For this review, take the finished solid that the model builds, in its own axes (mm). Give positions to 0.01 mm unless a question says otherwise; leave off trailing zeros. Use CSV: the item, a comma, the result in double quotes. Start each with the question number.
(1) Consider section A-A (y = -249.5). Give the number of separate pieces and of enclosed holes in the cut face, and give its area (3 significant figures).
(2) Clearance check with flat-ended pins moving along their axes: P1, Ø1.5, axis at x = 14.5, y = -333.5, coming from the -Z side; P2, Ø1.5, axis at y = -369, z = 14.5, coming from the -X side. State where each tip first meets the part, or that it passes through.
(3) Wall thickness on L1, parallel to Z at x = 7, y = -576.5; L2, parallel to Z at x = 10, y = -239.5 (3 decimals): over which ranges is each line inside the solid? List them lowest first. Write a range as from..to.
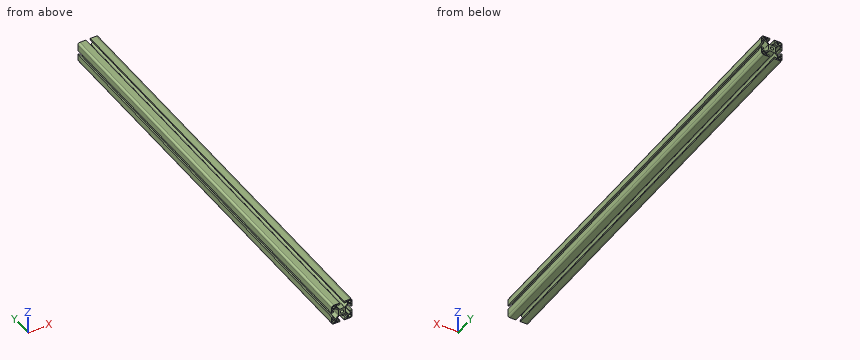
```python
from build123d import *

# Parameters (mm, degrees)
F0_R     = 2.45
F1_DEPTH = 460
F2_DEPTH = 160


# Not quite as in the source:
# - ends of sketch curves that miss each other by under 0.0002 mm in the source are joined


with BuildPart() as f1:
    # F0 (on Front) → F1 (new body)
    with BuildSketch(Plane.XZ):
        with BuildLine():
            Line((-3.1749674082, 15), (-12, 15))
            ThreePointArc((-12, 15), (-14.1213203436, 14.1213203436), (-15, 12))
            Line((-15, 12), (-15, 3.175))
            Line((-15, 3.175), (-13.0855346263, 3.175))
            ThreePointArc((-13.0855346263, 3.175), (-12.3835980145, 3.4627605788), (-12.0856407741, 4.1604300138))
            Line((-12.0856407741, 4.1604300138), (-12.0761692778, 4.8104300138))
            ThreePointArc((-12.0761692778, 4.8104300138), (-12.3638237087, 5.5269366118), (-13.0760631299, 5.825))
            Line((-13.0760631299, 5.825), (-13.5, 5.825))
            Line((-13.5, 5.825), (-13.5, 8.225))
            Line((-13.5, 8.225), (-9.8968845016, 8.225))
            ThreePointArc((-9.8968845016, 8.225), (-9.5279915195, 8.1544718757), (-9.2111331975, 7.9528359354))
            Line((-9.2111331975, 7.9528359354), (-5.4142486959, 4.3754933338))
            ThreePointArc((-5.4142486959, 4.3754933338), (-5.1819174045, 4.0440465354), (-5.1, 3.6476573984))
            Line((-5.1, 3.6476573984), (-5.1, -3.4999243287))
            ThreePointArc((-5.1, -3.4999243287), (-5.1782354607, -3.8876744211), (-5.4007002683, -4.2147528992))
            Line((-5.4007002683, -4.2147528992), (-9.2084959767, -7.9398285705))
            ThreePointArc((-9.2084959767, -7.9398285705), (-9.5301904718, -8.1509666761), (-9.9077957084, -8.225))
            Line((-9.9077957084, -8.225), (-13.5, -8.225))
            Line((-13.5, -8.225), (-13.5, -5.825))
            Line((-13.5, -5.825), (-13.0760631299, -5.825))
            ThreePointArc((-13.0760631299, -5.825), (-12.3638237087, -5.5269366118), (-12.0761692778, -4.8104300138))
            Line((-12.0761692778, -4.8104300138), (-12.0856407741, -4.1604300138))
            ThreePointArc((-12.0856407741, -4.1604300138), (-12.3835980145, -3.4627605788), (-13.0855346263, -3.175))
            Line((-13.0855346263, -3.175), (-15, -3.175))
            Line((-15, -3.175), (-15, -12))
            ThreePointArc((-15, -12), (-14.1213203436, -14.1213203436), (-12, -15))
            Line((-12, -15), (-3.175, -15))
            Line((-3.175, -15), (-3.175, -13.0855346263))
            ThreePointArc((-3.175, -13.0855346263), (-3.4627605788, -12.3835980145), (-4.1604300138, -12.0856407741))
            Line((-4.1604300138, -12.0856407741), (-4.8104300138, -12.0761692778))
            ThreePointArc((-4.8104300138, -12.0761692778), (-5.5269366118, -12.3638237087), (-5.825, -13.0760631299))
            Line((-5.825, -13.0760631299), (-5.825, -13.5))
            Line((-5.825, -13.5), (-8.225, -13.5))
            Line((-8.225, -13.5), (-8.225, -9.8968845016))
            ThreePointArc((-8.225, -9.8968845016), (-8.1544718757, -9.5279915195), (-7.9528359354, -9.2111331975))
            Line((-7.9528359354, -9.2111331975), (-4.3754933338, -5.4142486959))
            ThreePointArc((-4.3754933338, -5.4142486959), (-4.0440465354, -5.1819174045), (-3.6476573984, -5.1))
            Line((-3.6476573984, -5.1), (3.4999243287, -5.1))
            ThreePointArc((3.4999243287, -5.1), (3.8876744211, -5.1782354607), (4.2147528992, -5.4007002683))
            Line((4.2147528992, -5.4007002683), (7.9398285705, -9.2084959767))
            ThreePointArc((7.9398285705, -9.2084959767), (8.1509666761, -9.5301904718), (8.225, -9.9077957084))
            Line((8.225, -9.9077957084), (8.225, -13.5))
            Line((8.225, -13.5), (5.825, -13.5))
            Line((5.825, -13.5), (5.825, -13.0760631299))
            ThreePointArc((5.825, -13.0760631299), (5.5269366118, -12.3638237087), (4.8104300138, -12.0761692778))
            Line((4.8104300138, -12.0761692778), (4.1604300138, -12.0856407741))
            ThreePointArc((4.1604300138, -12.0856407741), (3.4627605788, -12.3835980145), (3.175, -13.0855346263))
            Line((3.175, -13.0855346263), (3.175, -15))
            Line((3.175, -15), (12, -15))
            ThreePointArc((12, -15), (14.1213203436, -14.1213203436), (15, -12))
            Line((15, -12), (15, -3.175))
            Line((15, -3.175), (13.0855346263, -3.175))
            ThreePointArc((13.0855346263, -3.175), (12.3835980145, -3.4627605788), (12.0856407741, -4.1604300138))
            Line((12.0856407741, -4.1604300138), (12.0761692778, -4.8104300138))
            ThreePointArc((12.0761692778, -4.8104300138), (12.3638237087, -5.5269366118), (13.0760631299, -5.825))
            Line((13.0760631299, -5.825), (13.5, -5.825))
            Line((13.5, -5.825), (13.5, -8.225))
            Line((13.5, -8.225), (9.9077957084, -8.225))
            ThreePointArc((9.9077957084, -8.225), (9.5301904718, -8.1509666761), (9.2084959767, -7.9398285705))
            Line((9.2084959767, -7.9398285705), (5.4007002683, -4.2147528992))
            ThreePointArc((5.4007002683, -4.2147528992), (5.1782354607, -3.8876744211), (5.1, -3.4999243287))
            Line((5.1, -3.4999243287), (5.1, 3.6476573984))
            ThreePointArc((5.1, 3.6476573984), (5.1819174045, 4.0440465354), (5.4142486959, 4.3754933338))
            Line((5.4142486959, 4.3754933338), (9.2111331975, 7.9528359354))
            ThreePointArc((9.2111331975, 7.9528359354), (9.5279915195, 8.1544718757), (9.8968845016, 8.225))
            Line((9.8968845016, 8.225), (13.5, 8.225))
            Line((13.5, 8.225), (13.5, 5.825))
            Line((13.5, 5.825), (13.0760631299, 5.825))
            ThreePointArc((13.0760631299, 5.825), (12.3638237087, 5.5269366118), (12.0761692778, 4.8104300138))
            Line((12.0761692778, 4.8104300138), (12.0856407741, 4.1604300138))
            ThreePointArc((12.0856407741, 4.1604300138), (12.3835980145, 3.4627605788), (13.0855346263, 3.175))
            Line((13.0855346263, 3.175), (15, 3.175))
            Line((15, 3.175), (15, 12))
            ThreePointArc((15, 12), (14.1213203436, 14.1213203436), (12, 15))
            Line((12, 15), (3.1750325918, 15))
            Line((3.1750325918, 15), (3.1750325918, 13.0854824722))
            ThreePointArc((3.1750325918, 13.0854824722), (3.4627931706, 12.3835458604), (4.1604626057, 12.0855886201))
            Line((4.1604626057, 12.0855886201), (4.8104626057, 12.0761171237))
            ThreePointArc((4.8104626057, 12.0761171237), (5.5269692036, 12.3637715546), (5.8250325918, 13.0760109758))
            Line((5.8250325918, 13.0760109758), (5.8250325918, 13.4999478459))
            Line((5.8250325918, 13.4999478459), (8.2250325918, 13.4999478459))
            Line((8.2250325918, 13.4999478459), (8.2250325918, 9.8968323476))
            ThreePointArc((8.2250325918, 9.8968323476), (8.1545044675, 9.5279393654), (7.9528685272, 9.2110810434))
            Line((7.9528685272, 9.2110810434), (4.3755259256, 5.4141965418))
            ThreePointArc((4.3755259256, 5.4141965418), (4.0440791272, 5.1818652505), (3.6476899902, 5.0999478459))
            Line((3.6476899902, 5.0999478459), (-3.4998917369, 5.0999478459))
            ThreePointArc((-3.4998917369, 5.0999478459), (-3.8876418293, 5.1781833067), (-4.2147203074, 5.4006481142))
            Line((-4.2147203074, 5.4006481142), (-7.9397959787, 9.2084438226))
            ThreePointArc((-7.9397959787, 9.2084438226), (-8.1509340843, 9.5301383177), (-8.2249674082, 9.9077435543))
            Line((-8.2249674082, 9.9077435543), (-8.2249674082, 13.4999478459))
            Line((-8.2249674082, 13.4999478459), (-5.8249674082, 13.4999478459))
            Line((-5.8249674082, 13.4999478459), (-5.8249674082, 13.0760109758))
            ThreePointArc((-5.8249674082, 13.0760109758), (-5.5269040199, 12.3637715546), (-4.810397422, 12.0761171237))
            Line((-4.810397422, 12.0761171237), (-4.160397422, 12.0855886201))
            ThreePointArc((-4.160397422, 12.0855886201), (-3.462727987, 12.3835458604), (-3.1749674082, 13.0854824722))
            Line((-3.1749674082, 13.0854824722), (-3.1749674082, 15))
        make_face()
        with BuildLine():
            Line((-13.5, -11.5), (-13.5, -9.7))
            Line((-13.5, -9.7), (-9.7, -9.7))
            Line((-9.7, -9.7), (-9.7, -13.5))
            Line((-9.7, -13.5), (-11.5, -13.5))
            ThreePointArc((-11.5, -13.5), (-12.9142135624, -12.9142135624), (-13.5, -11.5))
        make_face(mode=Mode.SUBTRACT)
        with BuildLine():
            Line((9.7, -9.7), (13.5, -9.7))
            Line((13.5, -9.7), (13.5, -11.5))
            ThreePointArc((13.5, -11.5), (12.9142135624, -12.9142135624), (11.5, -13.5))
            Line((11.5, -13.5), (9.7, -13.5))
            Line((9.7, -13.5), (9.7, -9.7))
        make_face(mode=Mode.SUBTRACT)
        with BuildLine():
            ThreePointArc((-13.5, 11.5), (-12.9142135624, 12.9142135624), (-11.5, 13.5))
            Line((-11.5, 13.5), (-9.7, 13.5))
            Line((-9.7, 13.5), (-9.7, 9.7))
            Line((-9.7, 9.7), (-13.5, 9.7))
            Line((-13.5, 9.7), (-13.5, 11.5))
        make_face(mode=Mode.SUBTRACT)
        Circle(F0_R, mode=Mode.SUBTRACT)
        with BuildLine():
            Line((9.7, 13.5), (11.5, 13.5))
            ThreePointArc((11.5, 13.5), (12.9142135624, 12.9142135624), (13.5, 11.5))
            Line((13.5, 11.5), (13.5, 9.7))
            Line((13.5, 9.7), (9.7, 9.7))
            Line((9.7, 9.7), (9.7, 13.5))
        make_face(mode=Mode.SUBTRACT)
    extrude(amount=F1_DEPTH)

    # F2 (add): a face of the model
    f2_faces = [f1.faces().sort_by_distance(p)[0] for p in [
        (5.2291627207, -460, 12.6659491494),
    ]]
    extrude(f2_faces, amount=F2_DEPTH)


solid = f1.part
```
Check result:
1,separate pieces,"1"
1,enclosed holes,"5"
1,area,"330 mm^2"
2,P1,"stops at z = -14.44"
2,P2,"stops at x = -14.44"
3,L1,"z = -15..-13.5, -8.25..-5.78, 5.87..8.2, 13.5..15"
3,L2,"z = -15..-13.5, -9.7..-8.225, 8.225..9.7, 13.5..15"
